```python
from build123d import *

# Parameters (mm, degrees)
F0_W     = 152.4
F0_H     = 50.8
F1_DEPTH = 76.2
F2_W     = 133.730998
F2_H     = 25.4
F3_DEPTH = 25.4
F4_W     = 133.730998
F4_H     = 25.4
F5_DEPTH = 25.4
F7_DEPTH = 25.4


with BuildPart() as f1:
    # F0 (on Front) → F1 (new body)
    with BuildSketch(Plane.XZ):
        with Locations((76.2, 25.4)):
            Rectangle(F0_W, F0_H)
    extrude(amount=-F1_DEPTH)

    # F2 (on face) → F3 (cut)
    with BuildSketch(Plane.XY.offset(50.8)):
        with Locations((85.534501, 12.7)):
            Rectangle(F2_W, F2_H)
    extrude(amount=-F3_DEPTH, mode=Mode.SUBTRACT)

    # F4 (on face) → F5 (cut)
    with BuildSketch(Plane.XY.offset(50.8)):
        with Locations((85.534501, 63.5)):
            Rectangle(F4_W, F4_H)
    extrude(amount=-F5_DEPTH, mode=Mode.SUBTRACT)

    # F6 (on face) → F7 (cut)
    with BuildSketch(Plane.XZ.offset(-25.4)):
        Polygon((152.4, 50.8), (18.669002, 50.8), (152.4, 25.4), align=None)
    extrude(amount=-F7_DEPTH, mode=Mode.SUBTRACT)


solid = f1.part
```
Could you check a few things on this model? Use its own coordinates, in mm. A direction names the side the tool comes from. Round coordinates to 2 decimals unless told otherwise and drop trailing zeros. Write each loop counter-clockwise with the first axis right and the second up, starting at its lowest first coordinate (ties: lowest second). Pieces come first, ordered by that corner, then holes. Notation, with made-up numbers: M 60.25,-30 L 119.25,-30 A21 cw 119.25,-20 Z; hole C 6,12 d11. An arc over 180 degrees is marked long. Write each question's results on one line, items separated by ' | '. Start each with the question number.
1. Imagine slicing it at D-D on y = 30. List the corners of the cut face in (x, z) for me, and give its area (3 significant figures).
2. Imagine slicing it at C-C on z = 45. List the corners of the cut face in (x, y) for me, and give its area (3 significant figures).
3. On a 3-axis mill with a long thin cutter (end or side, diameter ignored), from which of +Z, -Z, +X, -X, +Y, -Y can I reach the whole of each face in a straight line? I mean faces 1 (the face through (75, 76.2, 14)), 2 (the face through (85, 64, 25.4)), 3 (the face through (85, 13, 25.4)). Say none if no direction works.
4. Imagine slicing it at A-A on y = 60. List the corners of the cut face in (x, z) for me.
5. Imagine slicing it at B-B on x = 114. List the corners of the cut face in (y, z) for me, and give its area (3 significant figures).
6. I need wall thicknesses on L1, parallel to Z at x = 146, y = 5; L2, parallel to X at y = 17, z = 48.5; L3, parallel to Y at x = 61.5, z = 42.5. Which ranges of each line are inside material? Lowest first, please. Write a range as from..to.
7. I'm going to push flat-ended pins straight in: pin 1 Ø20.5 at (x, y) = (78.5, 14) entering from +Z; pin 2 Ø7.5 at (x, z) = (111, 32.5) entering from +Y; pin 3 Ø2 at (x, z) = (83, 31.5) entering from -Y. Where does each tip first touch, or does it pass through?
Result sheet:
1) outline: M 0,0 L 152.4,0 L 152.4,25.4 L 18.67,50.8 L 0,50.8 Z | area: 6,040 mm^2
2) outline: M 0,0 L 18.67,0 L 18.67,25.4 L 49.21,25.4 L 49.21,50.8 L 18.67,50.8 L 18.67,76.2 L 0,76.2 Z | area: 2,200 mm^2
3) face 1: +Z, -Z, +X, -X, +Y | face 2: +Z, +X, +Y | face 3: +Z, +X, -Y
4) outline: M 0,0 L 152.4,0 L 152.4,25.4 L 18.67,25.4 L 18.67,50.8 L 0,50.8 Z
5) outline: M 0,0 L 76.2,0 L 76.2,25.4 L 50.8,25.4 L 50.8,32.69 L 25.4,32.69 L 25.4,25.4 L 0,25.4 Z | area: 2,120 mm^2
6) L1: z = 0..25.4 | L2: x = 0..18.67 | L3: y = 25.4..50.8
7) pin 1: stops at z = 25.4 | pin 2: stops at y = 50.8 | pin 3: stops at y = 25.4
